from build123d import *

# Parameters (mm, degrees)
BOSS_EXTRUDE1_DEPTH = 8.75
SKETCH3_W           = 8
SKETCH3_H           = 16
CUT_EXTRUDE1_DEPTH  = 8.75
SKETCH4_W           = 84
SKETCH4_H           = 20
BOSS_EXTRUDE2_DEPTH = 3.75
BOSS_EXTRUDE3_DEPTH = 4.5
BOSS_EXTRUDE5_DEPTH = 4
SKETCH7_R           = 2.6
CUT_EXTRUDE2_DEPTH  = 14
CUT_EXTRUDE3_DEPTH  = 5
SKETCH10_R          = 1.6
SKETCH10_R_2        = 13
CUT_EXTRUDE4_DEPTH  = 5
SKETCH11_R          = 4.5
CUT_EXTRUDE5_DEPTH  = 5
SKETCH12_R          = 2.6
CUT_EXTRUDE6_DEPTH  = 3.75
SKETCH13_W          = 40
SKETCH13_H          = 9
BOSS_EXTRUDE6_DEPTH = 1
CUT_EXTRUDE14_DEPTH = 31
CUT_EXTRUDE15_DEPTH = 42
SKETCH17_W          = 40
SKETCH17_H          = 9
BOSS_EXTRUDE7_DEPTH = 1
CUT_EXTRUDE16_DEPTH = 10
CUT_EXTRUDE17_DEPTH = 40
SKETCH20_W          = 9
SKETCH20_H          = 20
BOSS_EXTRUDE8_DEPTH = 1
CUT_EXTRUDE19_DEPTH = 20
CUT_EXTRUDE20_DEPTH = 30
SKETCH23_R          = 2.6
CUT_EXTRUDE21_DEPTH = 1
SKETCH24_R          = 2.6
CUT_EXTRUDE22_DEPTH = 12
BOSS_EXTRUDE9_DEPTH = 3.75


with BuildPart() as part:
    # Sketch1 → Boss-Extrude1 (new body)
    with BuildSketch(Plane.XY):
        Polygon((0, 0), (0, 47), (69, 47), (84, 32), (84, 0), align=None)
    extrude(amount=BOSS_EXTRUDE1_DEPTH)

    # Sketch3 → Cut-Extrude1 (cut)
    with BuildSketch(Plane.XY.offset(8.75)):
        with Locations((70, 27)):
            Rectangle(SKETCH3_W, SKETCH3_H)
    extrude(amount=-CUT_EXTRUDE1_DEPTH, mode=Mode.SUBTRACT)

    # Sketch4 → Boss-Extrude2 (add)
    with BuildSketch(Plane.XZ):
        with Locations((42, 18.75)):
            Rectangle(SKETCH4_W, SKETCH4_H)
    extrude(amount=-BOSS_EXTRUDE2_DEPTH)

    # Sketch5 → Boss-Extrude3 (add)
    with BuildSketch(Plane.XZ):
        Polygon((60, -42.5), (56, -42.5), (13.5, 0), (60, 0), align=None)
    extrude(amount=-BOSS_EXTRUDE3_DEPTH)

    # Sketch6 → Boss-Extrude5 (add)
    with BuildSketch(Plane(origin=(60, 0, 0), x_dir=(0, 0, -1), z_dir=(1, 0, 0))):
        Polygon((0, 0), (0, 47), (38.5, 47), (42.5, 43), (42.5, 0), align=None)
    extrude(amount=-BOSS_EXTRUDE5_DEPTH)

    # Sketch7 → Cut-Extrude2 (cut)
    with BuildSketch(Plane(origin=(0, 0, 0), x_dir=(-1, 0, 0), z_dir=(0, 0, -1))):
        with Locations((-70, 14)):
            Circle(SKETCH7_R)
    extrude(amount=-CUT_EXTRUDE2_DEPTH, mode=Mode.SUBTRACT)

    # Sketch9 → Cut-Extrude3 (cut)
    with BuildSketch(Plane(origin=(0, 0, 0), x_dir=(-1, 0, 0), z_dir=(0, 0, -1))):
        Polygon((-84, 0), (-84, 32), (-69, 47), (-60, 47), (-60, 0), align=None)
    extrude(amount=-CUT_EXTRUDE3_DEPTH, mode=Mode.SUBTRACT)

    # Sketch10 → Cut-Extrude4 (cut)
    with BuildSketch(Plane(origin=(60, 0, 0), x_dir=(0, 0, -1), z_dir=(1, 0, 0))):
        with Locations((5.5, 42)):
            Circle(SKETCH10_R)
        with Locations((21, 26)):
            Circle(SKETCH10_R_2)
        with Locations((37, 41.5)):
            Circle(SKETCH10_R)
        with Locations((36.5, 10)):
            Circle(SKETCH10_R)
        with Locations((5, 10.5)):
            Circle(SKETCH10_R)
    extrude(amount=-CUT_EXTRUDE4_DEPTH, mode=Mode.SUBTRACT)

    # Sketch11 → Cut-Extrude5 (cut)
    with BuildSketch(Plane(origin=(0, 0, 0), x_dir=(-1, 0, 0), z_dir=(0, 0, -1))):
        with Locations((-50, 14)):
            Circle(SKETCH11_R)
        with Locations((-30, 14)):
            Circle(SKETCH11_R)
        with Locations((-10, 14)):
            Circle(SKETCH11_R)
        with Locations((-10, 34)):
            Circle(SKETCH11_R)
        with Locations((-30, 34)):
            Circle(SKETCH11_R)
    extrude(amount=-CUT_EXTRUDE5_DEPTH, mode=Mode.SUBTRACT)

    # Sketch12 → Cut-Extrude6 (cut)
    with BuildSketch(Plane(origin=(0, 0, 5), x_dir=(-1, 0, 0), z_dir=(0, 0, -1))):
        with Locations((-30, 34)):
            Circle(SKETCH12_R)
        with Locations((-10, 34)):
            Circle(SKETCH12_R)
        with Locations((-10, 14)):
            Circle(SKETCH12_R)
        with Locations((-30, 14)):
            Circle(SKETCH12_R)
        with Locations((-50, 14)):
            Circle(SKETCH12_R)
    extrude(amount=-CUT_EXTRUDE6_DEPTH, mode=Mode.SUBTRACT)

    # Sketch13 → Boss-Extrude6 (add)
    with BuildSketch(Plane.XY.offset(8.75)):
        with Locations((20, 34)):
            Rectangle(SKETCH13_W, SKETCH13_H)
        with Locations((20, 14)):
            Rectangle(SKETCH13_W, SKETCH13_H)
    extrude(amount=BOSS_EXTRUDE6_DEPTH)

    # Sketch16 → Cut-Extrude14 (cut)
    with BuildSketch(Plane(origin=(0, 38.5, 0), x_dir=(1, 0, 0), z_dir=(0, 1, 0))):
        Polygon((40, -8.75), (39, -9.75), (40, -9.75), align=None)
    extrude(amount=-CUT_EXTRUDE14_DEPTH, mode=Mode.SUBTRACT)

    # Sketch14 → Cut-Extrude15 (cut)
    with BuildSketch(Plane.ZY):
        Polygon((8.75, 38.5), (9.75, 37.5), (9.75, 38.5), align=None)
        Polygon((9.75, 29.5), (9.75, 30.502721412), (8.75, 29.5), align=None)
        Polygon((9.75, 18.5), (8.75, 18.5), (9.75, 17.5), align=None)
        Polygon((9.75, 9.5), (9.75, 10.5), (8.75, 9.5), align=None)
    extrude(amount=-CUT_EXTRUDE15_DEPTH, mode=Mode.SUBTRACT)

    # Sketch17 → Boss-Extrude7 (add)
    with BuildSketch(Plane(origin=(0, 3.75, 0), x_dir=(1, 0, 0), z_dir=(0, 1, 0))):
        with Locations((20, -18.75)):
            Rectangle(SKETCH17_W, SKETCH17_H)
    extrude(amount=BOSS_EXTRUDE7_DEPTH)

    # Sketch18 → Cut-Extrude16 (cut)
    with BuildSketch(Plane.XY.offset(23.25)):
        Polygon((40, 4.75), (39, 4.75), (40, 3.75), align=None)
    extrude(amount=-CUT_EXTRUDE16_DEPTH, mode=Mode.SUBTRACT)

    # Sketch19 → Cut-Extrude17 (cut)
    with BuildSketch(Plane.ZY):
        Polygon((14.25, 4.75), (14.25, 3.75), (15.25, 4.75), align=None)
        Polygon((23.25, 4.75), (23.25, 3.75), (22.25, 4.75), align=None)
    extrude(amount=-CUT_EXTRUDE17_DEPTH, mode=Mode.SUBTRACT)

    # Sketch20 → Boss-Extrude8 (add)
    with BuildSketch(Plane(origin=(0, 3.75, 0), x_dir=(1, 0, 0), z_dir=(0, 1, 0))):
        with Locations((50, -18.75)):
            Rectangle(SKETCH20_W, SKETCH20_H)
        with Locations((70, -18.75)):
            Rectangle(SKETCH20_W, SKETCH20_H)
    extrude(amount=BOSS_EXTRUDE8_DEPTH)

    # Sketch22 → Cut-Extrude19 (cut)
    with BuildSketch(Plane.XY.offset(28.75)):
        Polygon((45.5, 3.75), (45.5, 4.75), (46.5, 4.75), align=None)
        Polygon((54.5, 4.75), (54.5, 3.75), (53.5, 4.75), align=None)
        Polygon((65.5, 4.75), (66.5, 4.75), (65.5, 3.75), align=None)
        Polygon((74.5, 4.75), (74.5, 3.75), (73.5, 4.75), align=None)
    extrude(amount=-CUT_EXTRUDE19_DEPTH, mode=Mode.SUBTRACT)

    # Sketch21 → Cut-Extrude20 (cut)
    with BuildSketch(Plane.ZY.offset(-45.5)):
        Polygon((28.75, 3.75), (28.75, 4.75), (27.75, 4.75), align=None)
    extrude(amount=-CUT_EXTRUDE20_DEPTH, mode=Mode.SUBTRACT)

    # Sketch23 → Cut-Extrude21 (cut)
    with BuildSketch(Plane(origin=(0, 0, 8.75), x_dir=(-1, 0, 0), z_dir=(0, 0, -1))):
        with Locations((-30, 34)):
            Circle(SKETCH23_R)
        with Locations((-10, 34)):
            Circle(SKETCH23_R)
        with Locations((-30, 14)):
            Circle(SKETCH23_R)
        with Locations((-10, 14)):
            Circle(SKETCH23_R)
    extrude(amount=-CUT_EXTRUDE21_DEPTH, mode=Mode.SUBTRACT)

    # Sketch24 → Cut-Extrude22 (cut)
    with BuildSketch(Plane(origin=(0, 4.75, 0), x_dir=(1, 0, 0), z_dir=(0, 1, 0))):
        with Locations((10, -18.75)):
            Circle(SKETCH24_R)
        with Locations((30, -18.75)):
            Circle(SKETCH24_R)
        with Locations((50, -18.75)):
            Circle(SKETCH24_R)
        with Locations((70, -18.75)):
            Circle(SKETCH24_R)
    extrude(amount=-CUT_EXTRUDE22_DEPTH, mode=Mode.SUBTRACT)

    # Sketch25 → Boss-Extrude9 (add)
    with BuildSketch(Plane(origin=(84, 0, 0), x_dir=(0, 0, -1), z_dir=(1, 0, 0))):
        Polygon((-8.75, 23.75), (-28.75, 3.75), (-8.75, 3.75), align=None)
    extrude(amount=-BOSS_EXTRUDE9_DEPTH)


solid = part.part
Input: part model. Units: mm. Frame: model coordinates. A direction names the side the tool comes from. Give positions to 0.01 mm unless a question says otherwise; leave off trailing zeros. Write each loop counter-clockwise with the first axis right and the second up, starting at its lowest first coordinate (ties: lowest second). Pieces come first, ordered by that corner, then holes.
Q1. Set-up query: faces 1 (the face through (28, 12, 5)), 2 (the face through (56, 35, -31)), 3 (the face through (74, 27, 7)). Return all of +Z, -Z, +X, -X, +Y, -Y with unobstructed straight access to the full face (end or side cutting, diameter ignored); none if empty.
Q2. Section C-C, the plane x = 30. State how many separate pieces and enclosed holes the cut face has, plus the area to 3 significant figures.
Q3. Pull-direction query (Z, two-part tool) for faces 4 (the face through (60, 3.75, 19)), 5 (the face through (58.03, 40.58, -6.24)), 6 (the face through (48, 12, 5)), 7 (the face through (47.403, 2.408, 18.636)); classes: pulls with the +Z half, pulls with the -Z half, needs draft (parallel to the pull), parting line crosses it, or undercut.
Q4. Section A-A, the plane y = 26. Output: boundary loops of the cut face in (x, z).
Q5. First-contact query: P1, Ø8, axis at y = 38, z = -7, coming from the -X side; P2, Ø8, axis at x = 46.5, z = -18, coming from the +Y side; P3, Ø5.5, axis at x = 19, y = 12.5, coming from the +Z side. Flat tips, straight axial feed; report the tip coordinate or a pass-through.
Q6. Section D-D, the plane x = 16. Output: boundary loops of the cut face in (y, z).
Q7. Material intervals for probe 1 along Y at (x, z) = (30, 2); probe 2 along Z at (x, y) = (12, 23); probe 3 along X at (y, z) = (2, 18), sorted ascending.
Q8. Section B-B, the plane z = -16. Output: boundary loops of the cut face in (x, y), plus the area to 3 significant figures.
Filled in:
1. face 1: -Z
1. face 2: -Z, -X, +Y
1. face 3: +Z, -Z
2. separate pieces: 4
2. enclosed holes: 0
2. area: 420 mm2
3. face 4: needs draft
3. face 5: undercut
3. face 6: pulls with the -Z half
3. face 7: undercut
4. outline: (0, 0) - (56, 0) - (56, -8) - (60, -8) - (60, 5) - (66, 5) - (66, 8.75) - (0, 8.75) - close; (56, -42.5) - (60, -42.5) - (60, -34) - (56, -34) - close; (74, 5) - (84, 5) - (84, 8.75) - (74, 8.75) - close
5. P1: stops at x = 56
5. P2: stops at y = 4.5
5. P3: stops at z = 9.75
6. outline: (0, -2.5) - (4.5, -2.5) - (4.5, 0) - (47, 0) - (47, 8.75) - (38.5, 8.75) - (37.5, 9.75) - (30.5, 9.75) - (29.5, 8.75) - (18.5, 8.75) - (17.5, 9.75) - (10.5, 9.75) - (9.5, 8.75) - (3.75, 8.75) - (3.75, 14.25) - (4.75, 15.25) - (4.75, 22.25) - (3.75, 23.25) - (3.75, 28.75) - (0, 28.75) - close
7. probe 1: y = 0 to 9.5, 18.5 to 29.5, 38.5 to 47
7. probe 2: z = 0 to 8.75
7. probe 3: x = 0 to 7.51, 12.49 to 27.51, 32.49 to 47.51, 52.49 to 67.51, 72.49 to 84
8. outline: (29.5, 0) - (60, 0) - (60, 14) - (56, 14) - (56, 4.5) - (29.5, 4.5) - close; (56, 38) - (60, 38) - (60, 47) - (56, 47) - close
8. area: 211 mm2
